Geometry: see drawing. Coordinates: mm, zero at the bounding-box minimum. A direction names the side the tool comes from. Round coordinates to 2 decimals unless told otherwise and drop trailing zeros. Loops run counter-clockwise (first coordinate to the right, second up) from the corner with the lowest first, then second, coordinate; pieces in that order, holes last. Notation, with made-up numbers: (16.5, 28.25) - (66.5, 28.25) arc R12 cw to (66.5, 38.25) - close; hole circle Ø8 at (29, 44.25). An arc over 180 degrees is marked (long way). Use CSV: the item, a comma, the result in double quotes. Start each with the question number.
1. Cut plane C-C (z = 54). Return loops of the section in (x, y).
2. Cut plane A-A (x = 25). Give the number of separate pieces and of enclosed holes in the cut face.
3. Pin query (flat end, axial travel): P1, Ø8, axis at x = 33.5, z = 14.5, coming from the -Y side; P2, Ø8, axis at x = 24, y = 25, coming from the -Z side; P3, Ø1.5, axis at y = 12.5, z = 31.5, coming from the -X side (1 decimal). Return the tip coordinate at first contact, or that it passes through.
4. Material intervals for probe 1 along X at (y, z) = (24, 8) (1 decimal); probe 2 along Z at (x, y) = (25, 12) (1 decimal); probe 3 along Y at (x, z) = (25.5, 7), sorted ascending. Write a range as from..to.
5. Cut plane D-D (y = 17.5). Return loops of the section in (x, z) (1 decimal), and give its area (3 significant figures).
6. Cut plane B-B (y = 22). Return loops of the section in (x, z) (1 decimal).
7. Access query for the marked faces 1, 2 and 3. Directions: +Z, -Z, +X, -X, +Y, -Y. A direction counts if a zero-diameter tool reaches every point of the face in a straight line with its end or side. Return the directions, or none.
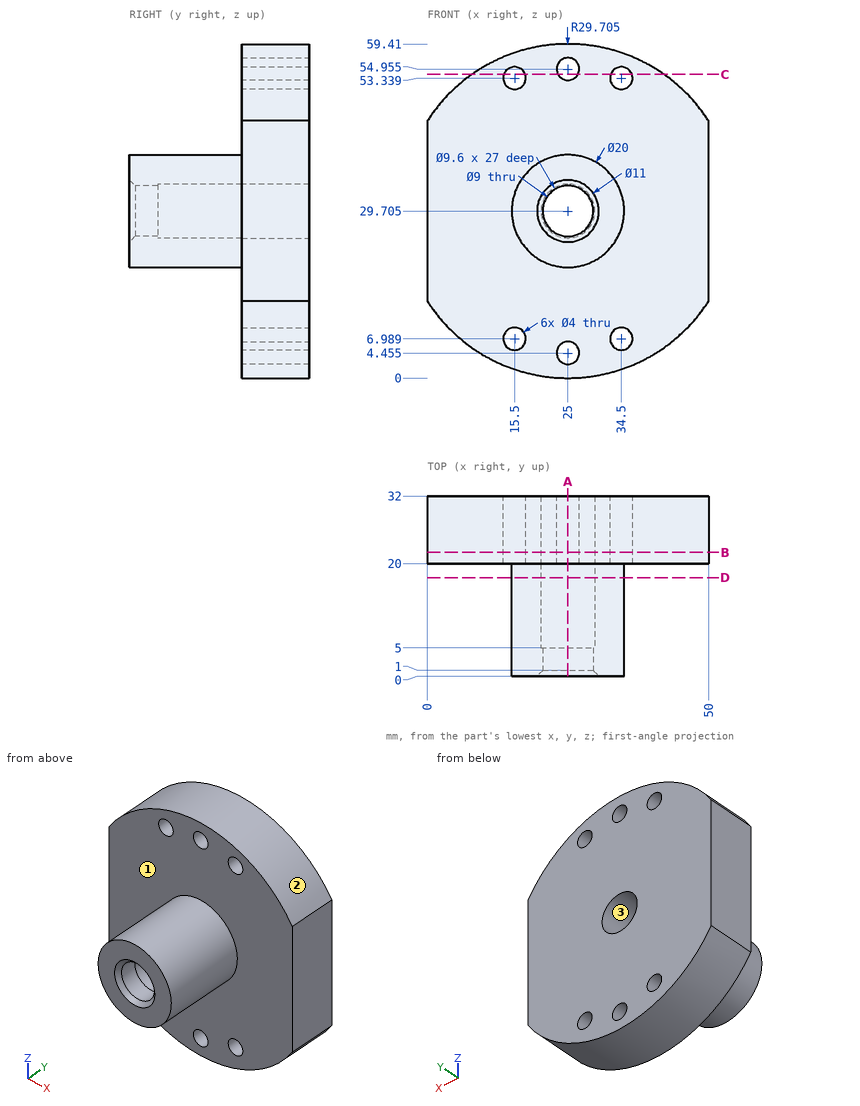
Established:
1,outline,"(7.91, 20) - (13.61, 20) - (13.61, 32) - (7.91, 32) - close; (17.39, 20) - (23.24, 20) - (23.24, 32) - (17.39, 32) - close; (26.76, 20) - (32.61, 20) - (32.61, 32) - (26.76, 32) - close; (36.39, 20) - (42.09, 20) - (42.09, 32) - (36.39, 32) - close"
2,separate pieces,"4"
2,enclosed holes,"0"
3,P1,"stops at y = 20"
3,P2,"stops at z = 0"
3,P3,"stops at x = 15.1"
4,probe 1,"x = 4.7..13.8, 17.2..32.8, 36.2..45.3"
4,probe 2,"z = 19.7..24.9, 34.5..39.7"
4,probe 3,"y = 20..32"
5,outline,"circle Ø20 at (25, 29.7); hole circle Ø9.6 at (25, 29.7)"
5,area,"242 mm2"
6,outline,"(0, 13.7) arc R29.7 ccw to (50, 13.7) - (50, 45.7) arc R29.7 ccw to (0, 45.7) - close; hole circle Ø4 at (15.5, 7); hole circle Ø4 at (15.5, 53.3); hole circle Ø9.6 at (25, 29.7); hole circle Ø4 at (25, 4.5); hole circle Ø4 at (25, 55); hole circle Ø4 at (34.5, 7); hole circle Ø4 at (34.5, 53.3)"
7,face 1,"-Y"
7,face 2,"+Z, +Y, -Y"
7,face 3,"+Y"
